For this review, use the dimensioned drawing (mm, ordinates from the lowest corner) and the shaded views. Round coordinates to 2 decimals unless told otherwise and drop trailing zeros. Order: outer loops, then holes, each group sorted by start corner. A loop starts at its lowest first (then second) coordinate and runs counter-clockwise, first axis right, second up. Notation, with made-up numbers: (-13.75, 34) -> (16.25, 34) arc R23 ccw to (16.25, 53) -> close; hole circle Ø1 at (0.5, -25.75). An arc over 180 degrees is marked (long way). Answer in a Markdown table with one row per item.
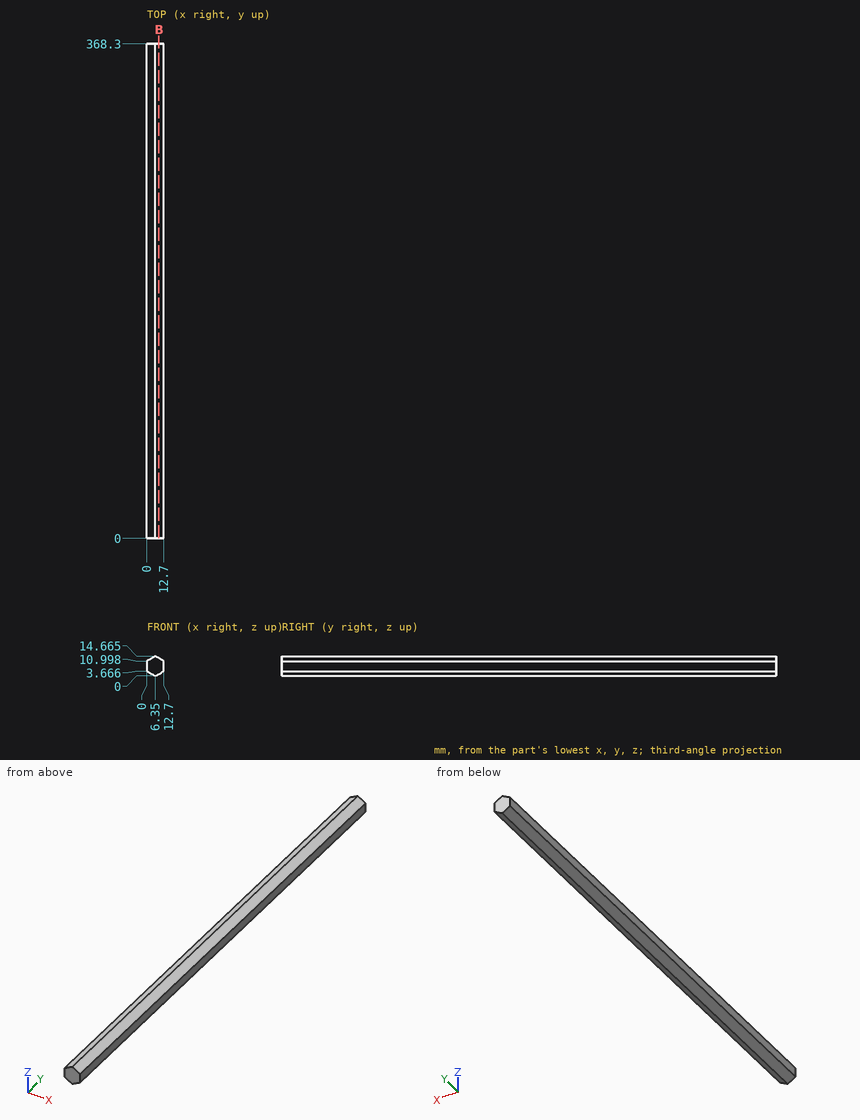
Q1. To check wall thickness, follow probe 1 along Z at (x, y) = (7, 29) (1 decimal); probe 2 along Z at (x, y) = (3.25, 107) (1 decimal); probe 3 along X at (y, z) = (122, 11.75) (1 decimal). State the ranges of each line that lie inside material, in increasing order.
Answer key:
| item | result |
|---|---|
| probe 1 | z = 0.4 to 14.3 |
| probe 2 | z = 1.8 to 12.9 |
| probe 3 | x = 1.3 to 11.4 |
Q2. Take a section at B-B, the plane x = 9. Write out the cut boundary in (y, z) (1 decimal).
Answer key:
| item | result |
|---|---|
| outline | (0, 1.5) -> (368.3, 1.5) -> (368.3, 13.1) -> (0, 13.1) -> close |
Q3. Clearance check with flat-ended pins moving along their axes: pin 1 Ø1.5 at (x, y) = (10, 247) entering from -Z (1 decimal); pin 2 Ø2 at (x, y) = (5, 320.5) entering from +Z; pin 3 Ø5 at (x, y) = (3, 81) entering from +Z (1 decimal). State where each tip first meets the part, or that it passes through.
Answer key:
| item | result |
|---|---|
| pin 1 | stops at z = 1.7 |
| pin 2 | stops at z = 14.46 |
| pin 3 | stops at z = 14.2 |
